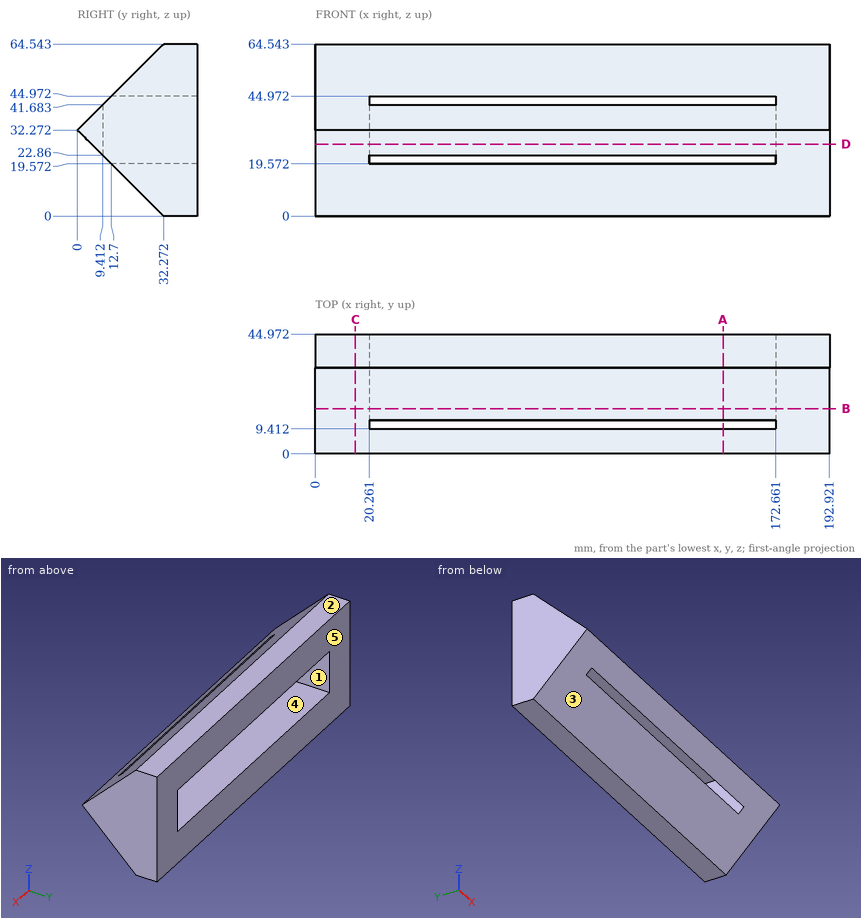
Could you check a few things on this drawing? It's one solid part, dimensions in mm from its lowest x, y, z. A direction names the side the tool comes from. Coordinates: 2 decimals unless noted, no trailing zeros. Loops run counter-clockwise (first coordinate to the right, second up) from the corner with the lowest first, then second, coordinate; pieces in that order, holes last.
1. I need wall thicknesses on L1, parallel to Z at x = 156.5, y = 40; L2, parallel to X at y = 11.5, z = 39; L3, parallel to Z at x = 29, y = 23. Which ranges of each line are inside material? Lowest first, please.
2. Imagine slicing it at D-D (z = 27). Please give me the cut outline in (x, y).
3. We'd pull the mould along Z, two halves only. Please class the marked faces 1, 2 and 3: released by +Z, released by -Z, zero draft, split by the parting line, or undercut.
4. Imagine slicing it at A-A (x = 153). Please give me the cut outline in (y, z), and give its area (3 significant figures).
5. Imagine slicing it at B-B (y = 17). Please give me the cut outline in (x, z), and give its area (3 significant figures).
6. For the marked faces 4 and 5, which set-ups out of +Z, -Z, +X, -X, +Y, -Y let a thin tool reach every point of the face, with its end or its side?
7. Imagine slicing it at C-C (x = 15). Please give me the cut outline in (y, z).
8. For P1, Ø12, axis at x = 111, z = 57.5, coming from the -Y side; P2, Ø3, axis at x = 155, y = 8.5, coming from the +Z side; P3, Ø1, axis at x = 110, z = 31.5, coming from the +Y side, each with a flat end and sliding along its axis, tell me the tip position at first contact or that it passes through.
Computed values:
1. L1: z = 0 to 19.57, 44.97 to 64.54
1. L2: x = 0 to 20.26, 172.66 to 192.92
1. L3: z = 9.27 to 19.57, 44.97 to 55.27
2. outline: (0, 5.27) - (192.92, 5.27) - (192.92, 44.97) - (172.66, 44.97) - (172.66, 9.41) - (20.26, 9.41) - (20.26, 44.97) - (0, 44.97) - close
3. face 1: undercut
3. face 2: released by +Z
3. face 3: released by -Z
4. outline: (0, 32.27) - (9.41, 22.86) - (9.41, 41.68) - close; (12.7, 19.57) - (32.27, 0) - (44.97, 0) - (44.97, 19.57) - close; (12.7, 44.97) - (44.97, 44.97) - (44.97, 64.54) - (32.27, 64.54) - close
4. area: 969 mm2
5. outline: (0, 15.27) - (192.92, 15.27) - (192.92, 49.27) - (0, 49.27) - close; hole (20.26, 19.57) - (172.66, 19.57) - (172.66, 44.97) - (20.26, 44.97) - close
5. area: 2,690 mm2
6. face 4: +Y, -Y
6. face 5: +Z, -Z, +X, -X, +Y
7. outline: (0, 32.27) - (32.27, 0) - (44.97, 0) - (44.97, 64.54) - (32.27, 64.54) - close
8. P1: stops at y = 19.23
8. P2: stops at z = 41.68
8. P3: stops at y = 9.41
